```python
from build123d import *

# Parameters (mm, degrees)
F0_W     = 221.488
F0_H     = 30.48
F0_W_2   = 34.29
F0_H_2   = 369.824
F1_DEPTH = 3
F2_W     = 86.36
F2_H     = 5.08
F2_R     = 2.5
F2_W_2   = 273.93447
F2_H_2   = 309.88
F2_W_3   = 6.35
F2_H_3   = 135
F2_R_2   = 3.81
F2_W_4   = 40.901455
F3_DEPTH = 25.4
F5_DEPTH = 25.4


with BuildPart() as f1:
    # F0 (on Front) → F1 (new body)
    with BuildSketch(Plane.XZ):
        Polygon((222.134481, 216.029425), (0.646481, 216.029425), (0.646481, 185.549425), (203.084481, 185.549425), (222.134481, 185.549425), align=None)
        with BuildLine():
            Line((203.084481, 185.549425), (0.646481, 185.549425))
            Line((0.646481, 185.549425), (0.646481, -235.074575))
            Line((0.646481, -235.074575), (222.134481, -235.074575))
            Line((222.134481, -235.074575), (228.484481, -235.074575))
            ThreePointArc((228.484481, -235.074575), (241.954865, -229.49496), (247.534481, -216.024575))
            Line((247.534481, -216.024575), (247.534481, -209.674575))
            Line((247.534481, -209.674575), (247.534481, 160.149425))
            Line((247.534481, 160.149425), (247.534481, 166.499425))
            ThreePointArc((247.534481, 166.499425), (241.954865, 179.969809), (228.484481, 185.549425))
            Line((228.484481, 185.549425), (222.134481, 185.549425))
            Line((222.134481, 185.549425), (203.084481, 185.549425))
        make_face()
        with Locations((111.390481, -250.314575)):
            Rectangle(F0_W, F0_H)
        with Locations((264.679481, -24.762575)):
            Rectangle(F0_W_2, F0_H_2)
    extrude(amount=F1_DEPTH)

    # F2 (on Front) → F3 (cut)
    with BuildSketch(Plane.XZ):
        Polygon((272.003669, -103.610899), (261.843669, -116.310899), (261.843669, -122.660899), (272.003669, -109.960899), align=None)
        Polygon((272.003669, -122.660899), (261.843669, -135.360899), (261.843669, -141.710899), (272.003669, -129.010899), align=None)
        Polygon((261.843669, -103.610899), (272.003669, -90.910899), (272.003669, -84.560899), (261.843669, -97.260899), align=None)
        Polygon((261.843669, -78.210899), (261.843669, -84.560899), (272.003669, -71.860899), (272.003669, -65.510899), align=None)
        Polygon((261.843669, -154.410899), (261.843669, -160.760899), (272.003669, -148.060899), (272.003669, -141.710899), align=None)
        Polygon((272.003669, -46.460899), (261.843669, -59.160899), (261.843669, -65.510899), (272.003669, -52.810899), align=None)
        Polygon((272.003669, -167.110899), (272.003669, -160.760899), (261.843669, -173.460899), (261.843669, -179.810899), align=None)
        Polygon((272.003669, -186.160899), (272.003669, -179.810899), (261.843669, -192.510899), (261.843669, -198.860899), align=None)
        with Locations((49.753669, -244.707899)):
            Rectangle(F2_W, F2_H)
        with Locations((49.753669, -253.597899)):
            Rectangle(F2_W, F2_H)
        with Locations((151.353669, -253.597899)):
            Rectangle(F2_W, F2_H)
        with Locations((151.353669, -244.707899)):
            Rectangle(F2_W, F2_H)
        with Locations((207.233669, -249.787899)):
            Circle(F2_R)
        with Locations((96.343246, 16.385425)):
            Rectangle(F2_W_2, F2_H_2)
        with Locations((272.299481, 32.649425)):
            Rectangle(F2_W_3, F2_H_3)
        with Locations((82.942481, 177.675425)):
            Circle(F2_R_2)
        with Locations((11.691753, 178.945425)):
            Rectangle(F2_W_4, F2_H)
        with Locations((239.660481, 15.728911)):
            Circle(F2_R_2)
        with Locations((0.646481, -144.904575)):
            Circle(F2_R_2)
    extrude(amount=F3_DEPTH, mode=Mode.SUBTRACT)

    # F4 (on Front) → F5 (cut)
    with BuildSketch(Plane.XZ):
        Polygon((155.873724, -202.75587), (213.023724, -153.22587), (206.673724, -153.22587), (149.523724, -202.75587), align=None)
        Polygon((155.873724, -219.26587), (232.073724, -153.22587), (225.723724, -153.22587), (149.523724, -219.26587), align=None)
        Polygon((155.873724, -188.551126), (196.633635, -153.22587), (190.283635, -153.22587), (149.523724, -188.551126), align=None)
        Polygon((173.147047, -153.22587), (149.523724, -173.699416), (155.873724, -173.699416), (179.497047, -153.22587), align=None)
        Polygon((194.59876, -219.26587), (232.073724, -186.787567), (225.723724, -186.787567), (188.24876, -219.26587), align=None)
        Polygon((225.723724, -170.842871), (169.851033, -219.26587), (176.201033, -219.26587), (232.073724, -170.842871), align=None)
        Polygon((225.723724, -201.960742), (205.756269, -219.26587), (212.106269, -219.26587), (232.073724, -201.960742), align=None)
    extrude(amount=F5_DEPTH, mode=Mode.SUBTRACT)


solid = f1.part
```
Could you check a few things on this model? Use its own coordinates, in mm. Round coordinates to 2 decimals unless told otherwise and drop trailing zeros. Order: outer loops, then holes, each group sorted by start corner. A loop starts at its lowest first (then second) coordinate and runs counter-clockwise, first axis right, second up. Notation, with made-up numbers: (-7.5, 10) -> (43.5, 10) arc R25 ccw to (43.5, 47) -> close; hole circle Ø5 at (-28.5, 18.25). An arc over 180 degrees is marked (long way). One line per question, with ' | ' between items.
Q1. If I drill on line 1 (X direction, y = -1.9, z = -242.5); line 2 (Z direction, x = 54, y = -1); line 3 (X direction, y = -1.1, z = -11.5), over which ranges is the centre line in solid material (lowest first)? Write a range as from..to.
Computed values:
line 1: 0.65..6.57, 92.93..108.17, 194.53..222.13 | line 2: -265.55..-256.14, -251.06..-247.25, -242.17..-138.55, 171.33..216.03 | line 3: 233.31..269.12, 275.47..281.82
Q2. If we section it at B-B on z = -29.5: Write out the boundary of the cut face in (x, y), plus the area to 3 significant figures.
Computed values:
outline: (233.31, -3) -> (269.12, -3) -> (269.12, 0) -> (233.31, 0) -> close; (275.47, -3) -> (281.82, -3) -> (281.82, 0) -> (275.47, 0) -> close | area: 126 mm²
Q3. If we section it at A-A on x = 47: Write out the boundary of the cut face in (y, z).
Computed values:
outline: (-3, -265.55) -> (0, -265.55) -> (0, -256.14) -> (-3, -256.14) -> close; (-3, -251.06) -> (0, -251.06) -> (0, -247.25) -> (-3, -247.25) -> close; (-3, -242.17) -> (0, -242.17) -> (0, -138.55) -> (-3, -138.55) -> close; (-3, 171.33) -> (0, 171.33) -> (0, 216.03) -> (-3, 216.03) -> close
Q4. If we section it at C-C on y = -2.1: Give the number of separate pieces and of enclosed holes in the cut face, plus the area to 3 significant figures.
Computed values:
separate pieces: 1 | enclosed holes: 23 | area: 52,600 mm²
Q5. I'm going to push flat-ended pins straight in: pin 1 (0.9 mm diameter, centred on y = -1, z = -244, fed in from +X); pin 2 (1.5 mm diameter, centred on y = -1, z = -125, fed in from -X); pin 3 (0.9 mm diameter, centred on x = 258, y = -1.5, fed in from +Z). Where does each tip first touch, or does it pass through?
Computed values:
pin 1: x = 222.13 | pin 2: x = 233.31 | pin 3: z = 160.15
Q6. We'd pull the mould along X, two halves only. Please class faces 1 (the face through (266.85, -1.48, -59.25)), 2 (the face through (241.81, -1.48, -229.64)), 3 (the face through (234, -3, -77)): released by +X, released by -X, zero draft, split by the parting line, or undercut.
Computed values:
face 1: undercut | face 2: released by +X | face 3: zero draft
